```python
from build123d import *

# Parameters (mm, degrees)
F0_W     = 417.5125
F0_H     = 6.35
F0_W_2   = 7.14375
F0_H_2   = 50.8
F0_H_3   = 17.4625
F0_H_4   = 7.14375
F0_W_3   = 6.35
F0_H_5   = 9.525
F1_DEPTH = 6.35
F2_DEPTH = 3.175


with BuildPart() as f1:
    # F0 (on Top) → F1 (new body)
    with BuildSketch(Plane.XY):
        with Locations((0, 49.2125)):
            Rectangle(F0_W, F0_H)
        with Locations((0, -49.2125)):
            Rectangle(F0_W, F0_H)
        with Locations((-212.328125, -11.1125)):
            Rectangle(F0_W_2, F0_H_2)
        with Locations((-212.328125, 30.1625)):
            Rectangle(F0_W_2, F0_H_3)
        with Locations((0, 42.465625)):
            Rectangle(F0_W, F0_H_4)
        with Locations((0, 17.859375)):
            Rectangle(F0_W, F0_H_4)
        Polygon((222.25, -52.3875), (222.25, 52.3875), (215.9, 52.3875), (215.9, 46.0375), (215.9, 38.89375), (215.9, 21.43125), (215.9, 14.2875), (215.9, -36.5125), (215.9, -46.0375), (215.9, -52.3875), align=None)
        with Locations((-219.075, -11.1125)):
            Rectangle(F0_W_3, F0_H_2)
        with Locations((0, -41.275)):
            Rectangle(F0_W, F0_H_5)
        with Locations((0, -11.1125)):
            Rectangle(F0_W, F0_H_2)
        with Locations((0, 30.1625)):
            Rectangle(F0_W, F0_H_3)
        with Locations((-219.075, 42.465625)):
            Rectangle(F0_W_3, F0_H_4)
        with Locations((-212.328125, 49.2125)):
            Rectangle(F0_W_2, F0_H)
        with Locations((212.328125, 49.2125)):
            Rectangle(F0_W_2, F0_H)
        with Locations((-219.075, 49.2125)):
            Rectangle(F0_W_3, F0_H)
        with Locations((-212.328125, 17.859375)):
            Rectangle(F0_W_2, F0_H_4)
        with Locations((-212.328125, 42.465625)):
            Rectangle(F0_W_2, F0_H_4)
        with Locations((212.328125, 30.1625)):
            Rectangle(F0_W_2, F0_H_3)
        with Locations((-219.075, 30.1625)):
            Rectangle(F0_W_3, F0_H_3)
        with Locations((-219.075, 17.859375)):
            Rectangle(F0_W_3, F0_H_4)
        with Locations((-219.075, -41.275)):
            Rectangle(F0_W_3, F0_H_5)
        with Locations((212.328125, -41.275)):
            Rectangle(F0_W_2, F0_H_5)
        with Locations((212.328125, 42.465625)):
            Rectangle(F0_W_2, F0_H_4)
        with Locations((212.328125, 17.859375)):
            Rectangle(F0_W_2, F0_H_4)
        with Locations((-212.328125, -41.275)):
            Rectangle(F0_W_2, F0_H_5)
        with Locations((-219.075, -49.2125)):
            Rectangle(F0_W_3, F0_H)
        with Locations((212.328125, -11.1125)):
            Rectangle(F0_W_2, F0_H_2)
    extrude(amount=-F1_DEPTH)

    # F0 (on Top) → F2 (cut)
    with BuildSketch(Plane.XY):
        with Locations((-212.328125, -41.275)):
            Rectangle(F0_W_2, F0_H_5)
        with Locations((-212.328125, -11.1125)):
            Rectangle(F0_W_2, F0_H_2)
        with Locations((-212.328125, 17.859375)):
            Rectangle(F0_W_2, F0_H_4)
        with Locations((-212.328125, 30.1625)):
            Rectangle(F0_W_2, F0_H_3)
        with Locations((-212.328125, 42.465625)):
            Rectangle(F0_W_2, F0_H_4)
        with Locations((-212.328125, 49.2125)):
            Rectangle(F0_W_2, F0_H)
        with Locations((-219.075, 42.465625)):
            Rectangle(F0_W_3, F0_H_4)
        with Locations((-219.075, 17.859375)):
            Rectangle(F0_W_3, F0_H_4)
        with Locations((0, 17.859375)):
            Rectangle(F0_W, F0_H_4)
        with Locations((0, 42.465625)):
            Rectangle(F0_W, F0_H_4)
        with Locations((-219.075, -41.275)):
            Rectangle(F0_W_3, F0_H_5)
        with Locations((0, -41.275)):
            Rectangle(F0_W, F0_H_5)
        with Locations((212.328125, -41.275)):
            Rectangle(F0_W_2, F0_H_5)
        with Locations((212.328125, 17.859375)):
            Rectangle(F0_W_2, F0_H_4)
        with Locations((212.328125, 42.465625)):
            Rectangle(F0_W_2, F0_H_4)
        with Locations((212.328125, 49.2125)):
            Rectangle(F0_W_2, F0_H)
        with Locations((212.328125, 30.1625)):
            Rectangle(F0_W_2, F0_H_3)
        with Locations((212.328125, -11.1125)):
            Rectangle(F0_W_2, F0_H_2)
    extrude(amount=-F2_DEPTH, mode=Mode.SUBTRACT)


solid = f1.part
```
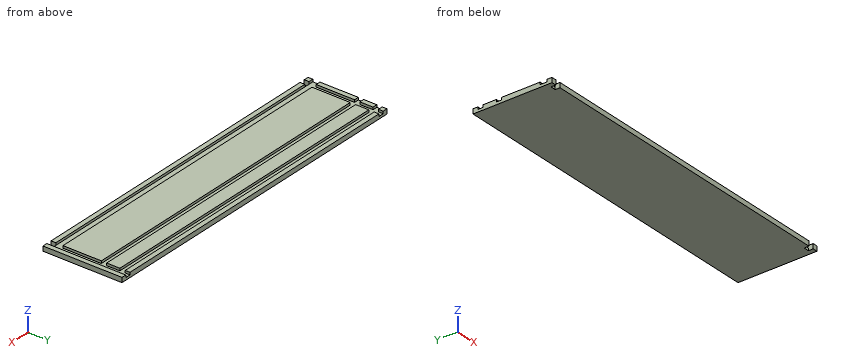
Could you check a few things on this model? Use its own coordinates, in mm. Coordinates: 2 decimals unless noted, no trailing zeros. Write each loop counter-clockwise with the first axis right and the second up, starting at its lowest first coordinate (ties: lowest second). Pieces come first, ordered by that corner, then holes. Notation, with made-up numbers: M -13,-39.5 L 28,-39.5 A18 cw 28,-23.5 Z; hole C 17.5,27 d8. An arc over 180 degrees is marked long. Answer as CSV lines item,"result". Start each with the question number.
1) I want a section at D-D, the plane y = -40.5. Please give me the cut outline in (x, z) (3 decimals).
2) I want a section at B-B, the plane y = -18.5. Please give me the cut outline in (x, z) (3 decimals), and give its area (3 significant figures).
3) I want a section at C-C, the plane z = -1.5. Give the number of separate pieces and of enclosed holes in the cut face, and give its area (3 significant figures).
4) Please list where these lines run through material, in increasing order: line 1 (X direction, y = -20.5, z = -1.25); line 2 (Y direction, x = 42, z = -1); line 3 (Z direction, x = -7, y = -40) (3 decimals). Write a range as from..to.
5) For P1, Ø1.6, axis at x = 213, z = -4.5, coming from the -Y side; P2, Ø1.5, axis at x = -109.5, y = 20, coming from the +Z side (3 decimals), each with a flat end and sliding along its axis, tell me the tip position at first contact or that it passes through.
Data:
1,outline,"M -222.25,-6.35 L 222.25,-6.35 L 222.25,0 L 215.9,0 L 215.9,-3.175 L -222.25,-3.175 Z"
2,outline,"M -222.25,-6.35 L 222.25,-6.35 L 222.25,0 L 215.9,0 L 215.9,-3.175 L 208.756,-3.175 L 208.756,0 L -208.756,0 L -208.756,-3.175 L -215.9,-3.175 L -215.9,0 L -222.25,0 Z"
2,area,"2,780 mm^2"
3,separate pieces,"9"
3,enclosed holes,"0"
3,area,"35,000 mm^2"
4,line 1,"x = -222.25..-215.9, -208.76..208.76, 215.9..222.25"
4,line 2,"y = -52.39..-46.04, -36.51..14.29, 21.43..38.89, 46.04..52.39"
4,line 3,"z = -6.35..-3.175"
5,P1,"stops at y = -46.04"
5,P2,"stops at z = -3.175"
